from build123d import *

# Parameters (mm, degrees)
CROQUIS2_W              = 34.5
CROQUIS2_H              = 18
SALIENTE_EXTRUIR1_DEPTH = 1.5
CROQUIS3_R              = 0.5
CORTAR_EXTRUIR1_DEPTH   = 1.5


with BuildPart() as part:
    # Croquis2 → Saliente-Extruir1 (new body)
    with BuildSketch(Plane.XY):
        with Locations((17.25, 9)):
            Rectangle(CROQUIS2_W, CROQUIS2_H)
    extrude(amount=SALIENTE_EXTRUIR1_DEPTH)

    # Croquis3 → Cortar-Extruir1 (cut)
    with BuildSketch(Plane.XY.offset(1.5)):
        with Locations((4.02, 2.47)):
            Circle(CROQUIS3_R)
        with Locations((1.47, 2.47)):
            Circle(CROQUIS3_R)
        with Locations((1.5, 12.96)):
            Circle(CROQUIS3_R)
        with Locations((1.5, 10.42)):
            Circle(CROQUIS3_R)
        with Locations((1.5, 7.88)):
            Circle(CROQUIS3_R)
        with Locations((1.5, 5.34)):
            Circle(CROQUIS3_R)
        with Locations((6.57, 2.47)):
            Circle(CROQUIS3_R)
        with Locations((9.12, 2.47)):
            Circle(CROQUIS3_R)
        with Locations((11.67, 2.47)):
            Circle(CROQUIS3_R)
        with Locations((14.22, 2.47)):
            Circle(CROQUIS3_R)
        with Locations((16.77, 2.47)):
            Circle(CROQUIS3_R)
        with Locations((19.32, 2.47)):
            Circle(CROQUIS3_R)
        with Locations((21.87, 2.47)):
            Circle(CROQUIS3_R)
        with Locations((24.42, 2.47)):
            Circle(CROQUIS3_R)
        with Locations((26.97, 2.47)):
            Circle(CROQUIS3_R)
        with Locations((29.52, 2.47)):
            Circle(CROQUIS3_R)
        with Locations((4.02, 15.47)):
            Circle(CROQUIS3_R)
        with Locations((6.57, 15.47)):
            Circle(CROQUIS3_R)
        with Locations((9.12, 15.47)):
            Circle(CROQUIS3_R)
        with Locations((11.67, 15.47)):
            Circle(CROQUIS3_R)
        with Locations((14.22, 15.47)):
            Circle(CROQUIS3_R)
        with Locations((16.77, 15.47)):
            Circle(CROQUIS3_R)
        with Locations((19.32, 15.47)):
            Circle(CROQUIS3_R)
        with Locations((21.87, 15.47)):
            Circle(CROQUIS3_R)
        with Locations((24.42, 15.47)):
            Circle(CROQUIS3_R)
        with Locations((26.97, 15.47)):
            Circle(CROQUIS3_R)
        with Locations((29.52, 15.47)):
            Circle(CROQUIS3_R)
        with Locations((1.47, 15.47)):
            Circle(CROQUIS3_R)
        with Locations((32.44, 12.96)):
            Circle(CROQUIS3_R)
        with Locations((32.44, 10.42)):
            Circle(CROQUIS3_R)
        with Locations((32.44, 7.88)):
            Circle(CROQUIS3_R)
        with Locations((15.43, 13.5)):
            Circle(CROQUIS3_R)
        with Locations((12.89, 13.5)):
            Circle(CROQUIS3_R)
    extrude(amount=-CORTAR_EXTRUIR1_DEPTH, mode=Mode.SUBTRACT)


solid = part.part
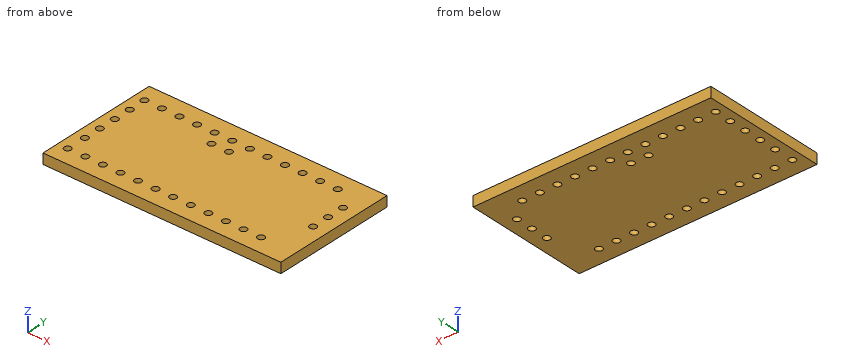
Input: part model. Units: mm. Frame: model coordinates. Round coordinates to 2 decimals unless told otherwise and drop trailing zeros. Order: outer loops, then holes, each group sorted by start corner. A loop starts at its lowest first (then second) coordinate and runs counter-clockwise, first axis right, second up. Notation, with made-up numbers: (79, 86) - (136, 86) arc R5 cw to (136, 93) - close; hole circle Ø5 at (-32.5, -34.5). An arc over 180 degrees is marked (long way). Answer as a JSON object with one key per item and string values. Group by question number.
(1) Cut plane D-D (x = 15.43). Return loops of the section in (y, z).
(2) Cut plane C-C (x = 1.5). Return loops of the section in (y, z), then the cut area to 3 significant figures.
(3) Cut plane B-B (y = 5.34). Return loops of the section in (x, z), then the cut area to 4 significant figures.
(4) Material intervals for probe 1 along Y at (x, z) = (29.5, 0.85); probe 2 along Y at (x, z) = (32, 1.15); probe 3 along X at (y, z) = (10.75, 0.6), sorted ascending. Write a range as from..to.
(5) Cut plane A-A (x = 11.67). Return loops of the section in (y, z), then the cut area to 3 significant figures.
Here are the results:
{
 "1": {"outline": "(0, 0) - (13, 0) - (13, 1.5) - (0, 1.5) - close; (14, 0) - (18, 0) - (18, 1.5) - (14, 1.5) - close"},
 "2": {"outline": "(0, 0) - (1.97, 0) - (1.97, 1.5) - (0, 1.5) - close; (2.97, 0) - (4.84, 0) - (4.84, 1.5) - (2.97, 1.5) - close; (5.84, 0) - (7.38, 0) - (7.38, 1.5) - (5.84, 1.5) - close; (8.38, 0) - (9.92, 0) - (9.92, 1.5) - (8.38, 1.5) - close; (10.92, 0) - (12.46, 0) - (12.46, 1.5) - (10.92, 1.5) - close; (13.46, 0) - (14.97, 0) - (14.97, 1.5) - (13.46, 1.5) - close; (15.97, 0) - (18, 0) - (18, 1.5) - (15.97, 1.5) - close", "area": "18.0 mm^2"},
 "3": {"outline": "(0, 0) - (1, 0) - (1, 1.5) - (0, 1.5) - close; (2, 0) - (34.5, 0) - (34.5, 1.5) - (2, 1.5) - close", "area": "50.25 mm^2"},
 "4": {"probe 1": "y = 0..1.97, 2.97..14.97, 15.97..18", "probe 2": "y = 0..7.64, 8.12..10.18, 10.66..12.72, 13.2..18", "probe 3": "x = 0..1.12, 1.88..32.06, 32.82..34.5"},
 "5": {"outline": "(0, 0) - (1.97, 0) - (1.97, 1.5) - (0, 1.5) - close; (2.97, 0) - (14.97, 0) - (14.97, 1.5) - (2.97, 1.5) - close; (15.97, 0) - (18, 0) - (18, 1.5) - (15.97, 1.5) - close", "area": "24.0 mm^2"}
}
